The figure shows three views and two pictorial views of one solid part (mm, origin at its lowest corner). Answer the questions. A direction names the side the tool comes from. Coordinates: 2 decimals unless noted, no trailing zeros. Loops run counter-clockwise (first coordinate to the right, second up) from the corner with the lowest first, then second, coordinate; pieces in that order, holes last.
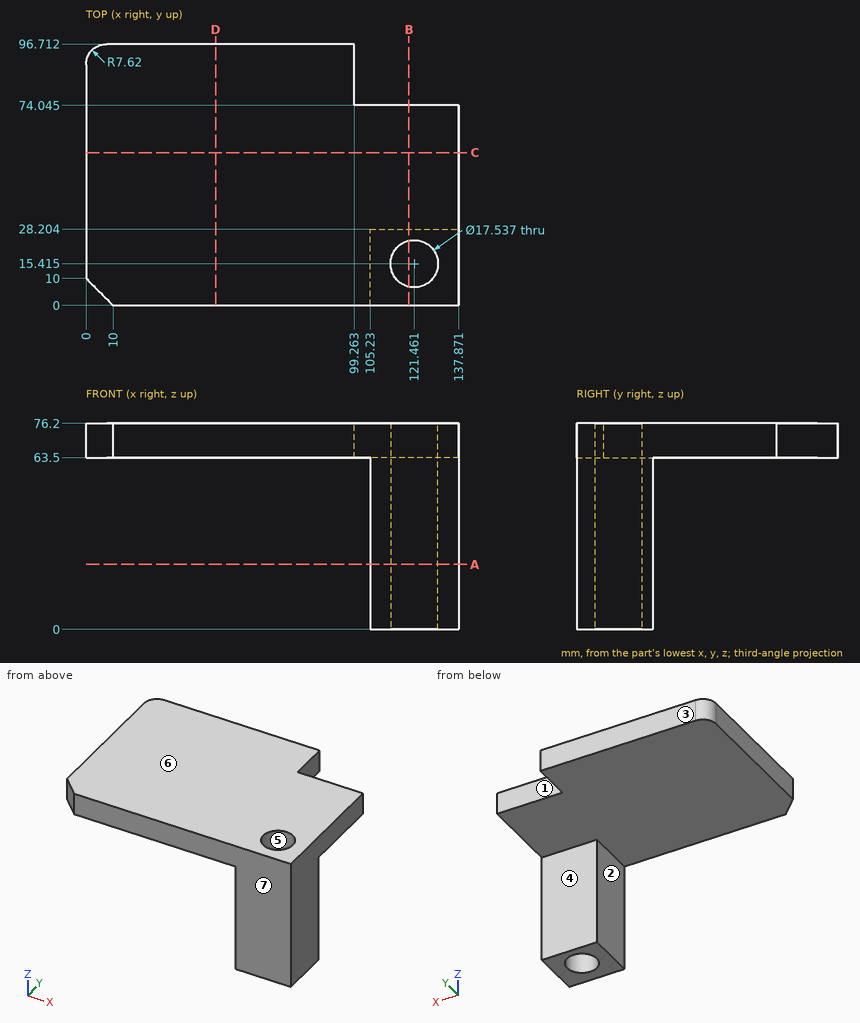
Q1. A cutting plane is placed at A-A (z = 24). Give the vertices of the cut face in (x, y) (1 decimal).
Findings below:
outline: (105.2, 0) - (137.9, 0) - (137.9, 28.2) - (105.2, 28.2) - close; hole circle Ø17.5 at (121.5, 15.4)
Q2. A cutting plane is placed at C-C (y = 56.5). Give the vertices of the cut face in (x, z).
Findings below:
outline: (0, 63.5) - (137.87, 63.5) - (137.87, 76.2) - (0, 76.2) - close
Q3. A cutting plane is placed at D-D (x = 48). Give the vertices of the cut face in (y, z), then the cut area to 3 significant figures.
Findings below:
outline: (0, 63.5) - (96.71, 63.5) - (96.71, 76.2) - (0, 76.2) - close
area: 1,230 mm2
Q4. Which of the six approach directions +Z, -Z, +X, -X, +Y, -Y give full straight-line access (tool end or side, diameter ignored) to the marked faces 1, 2 and 3?
Findings below:
face 1: +Z, -Z, +X, +Y
face 2: -Z, -X, +Y, -Y
face 3: +Z, -Z, +X, -X, +Y
Q5. Determine the mould class of the marked faces 4, 5, 6 and 7 for opening direction Y: +Y half, -Y half, draft (parallel to the pull), parting line (faces both ways), or undercut.
Findings below:
face 4: +Y half
face 5: undercut
face 6: draft
face 7: -Y half
Q6. A cutting plane is placed at B-B (x = 119.5). Give the vertices of the cut face in (y, z) (1 decimal), then the cut area to 3 significant figures.
Findings below:
outline: (0, 0) - (6.9, 0) - (6.9, 76.2) - (0, 76.2) - close; (24, 0) - (28.2, 0) - (28.2, 63.5) - (74, 63.5) - (74, 76.2) - (24, 76.2) - close
area: 1,430 mm2
Q7. Flat-ended cylindrical pins translate along their axes: pin 1 Ø1 at (x, y) = (52.5, 49) entering from -Z; pin 2 Ø1 at (y, z) = (21.5, 45.5) entering from -X; pin 3 Ø14 at (x, z) = (119.5, 72.5) entering from +Y (1 decimal); pin 4 Ø16 at (x, y) = (121.46, 15.42) entering from +Z. Find the tip coordinate at first contact, or state that the pin passes through.
Findings below:
pin 1: stops at z = 63.5
pin 2: stops at x = 105.23
pin 3: stops at y = 74
pin 4: passes through
Q8. Straight lines are drawn through the part: probe 1 along X at (y, z) = (15.5, 68.5); probe 2 along Z at (x, y) = (85.5, 66.5); probe 3 along Y at (x, z) = (126.5, 43) (1 decimal). For each, find the intervals that lie inside material, in ascending order.
Findings below:
probe 1: x = 0 to 112.69, 130.23 to 137.87
probe 2: z = 63.5 to 76.2
probe 3: y = 0 to 8.2, 22.6 to 28.2
